CAD build for the part. Positions are in the model's coordinates, mm. A direction names the side the tool comes from. Give positions to 0.01 mm unless a question says otherwise; leave off trailing zeros. Write each loop counter-clockwise with the first axis right and the second up, starting at its lowest first coordinate (ties: lowest second). Pieces come first, ordered by that corner, then holes. Notation, with made-up numbers: (54, 57) - (58, 57) arc R10 cw to (58, 64) - close; hole circle Ø9 at (44.25, 37.5). An arc over 180 degrees is marked (long way). Answer as a JSON object with one key per item and string values.
from build123d import *

# Parameters (mm, degrees)
SKETCH_1_W          = 15
SKETCH_1_H          = 10
SKETCH_1_W_2        = 13
SKETCH_1_H_2        = 8
EXTRUDE_1_DEPTH     = 182.5
SKETCH_2_R          = 2.1
CUT_EXTRUDE_1_DEPTH = 183.927581299
SKETCH_3_R          = 1.6
SKETCH_3_R_2        = 2.1
CUT_EXTRUDE_2_DEPTH = 184.183651017


with BuildPart() as part:
    # ｽｹｯﾁ1 → 押し出し-薄板1 (new body)
    with BuildSketch(Plane(origin=(0, 0, 0), x_dir=(1, 0, 0), z_dir=(0, 1, 0))):
        Rectangle(SKETCH_1_W, SKETCH_1_H)
        Rectangle(SKETCH_1_W_2, SKETCH_1_H_2, mode=Mode.SUBTRACT)
    extrude(amount=EXTRUDE_1_DEPTH)

    # ｽｹｯﾁ2 → ｶｯﾄ - 押し出し1 (cut, through all)
    with BuildSketch(Plane.XY.offset(5)):
        with Locations((0, 7.5)):
            Circle(SKETCH_2_R)
        with Locations((0, 65)):
            Circle(SKETCH_2_R)
        with Locations((0, 157.5)):
            Circle(SKETCH_2_R)
        with Locations((0, 177.5)):
            Circle(SKETCH_2_R)
    extrude(amount=-CUT_EXTRUDE_1_DEPTH, mode=Mode.SUBTRACT)

    # ｽｹｯﾁ3 → ｶｯﾄ - 押し出し2 (cut, through all)
    with BuildSketch(Plane(origin=(7.5, 0, 0), x_dir=(0, 0, -1), z_dir=(1, 0, 0))):
        with Locations((0, 20)):
            Circle(SKETCH_3_R)
        with Locations((0, 60)):
            Circle(SKETCH_3_R_2)
        with Locations((0, 40)):
            Circle(SKETCH_3_R)
    extrude(amount=-CUT_EXTRUDE_2_DEPTH, mode=Mode.SUBTRACT)


solid = part.part
Item 1: Mould opens along Z. For faces 3 (the cylindrical face through (-1.666, 63.722, 4.507)), 4 (the cylindrical face through (7.01, 57.95, 0.46)), 5 (the flat face through (0, 90, -5)) say: +Z half, -Z half, draft (parallel to the pull), parting line (faces both ways), or undercut.
Entries:
{"face 3": "draft", "face 4": "undercut", "face 5": "-Z half"}
Item 2: Which spindle directions (+Z, -Z, +X, -X, +Y, -Y) get a long thin tool onto all of the face, cutting with end or side? Do faces 1 (the cylindrical face through (-0.273, 179.582, -4.493)), 2 (the flat face through (0, 90, 4)). Say none if no direction does.
Entries:
{"face 1": "+Z, -Z", "face 2": "+Y, -Y"}
Item 3: Cut at B-B (y = 88). Give the cut face in (x, z), and give its area (3 significant figures).
Entries:
{"outline": "(-7.5, -5) - (7.5, -5) - (7.5, 5) - (-7.5, 5) - close; hole (-6.5, -4) - (6.5, -4) - (6.5, 4) - (-6.5, 4) - close", "area": "46.0 mm2"}
Item 4: Cut at A-A (x = -4.25). Give the cut face in (y, z).
Entries:
{"outline": "(0, -5) - (182.5, -5) - (182.5, -4) - (0, -4) - close; (0, 4) - (182.5, 4) - (182.5, 5) - (0, 5) - close"}
Item 5: Cut at D-D (y = 65). Give the cut face in (x, z).
Entries:
{"outline": "(-7.5, -5) - (-2.1, -5) - (-2.1, -4) - (-6.5, -4) - (-6.5, 4) - (-2.1, 4) - (-2.1, 5) - (-7.5, 5) - close; (2.1, -5) - (7.5, -5) - (7.5, 5) - (2.1, 5) - (2.1, 4) - (6.5, 4) - (6.5, -4) - (2.1, -4) - close"}
Item 6: Cut at C-C (z = 0). State how many separate pieces and enclosed holes the cut face has, and give its area (3 significant figures).
Entries:
{"separate pieces": "8", "enclosed holes": "0", "area": "344 mm2"}
Item 7: Probe line 1 (Y direction, x = 0, z = 4.65); line 2 (X direction, y = 145.5, z = -2.75); line 3 (Z direction, x = -5.75, y = 84). List the from-to ranges inside material, lowest first. Write a range as from..to.
Entries:
{"line 1": "0..5.4, 9.6..62.9, 67.1..155.4, 159.6..175.4, 179.6..182.5", "line 2": "-7.5..-6.5, 6.5..7.5", "line 3": "-5..-4, 4..5"}
